from build123d import *

# Parameters (mm, degrees)
F1_DEPTH = 4.65
F2_R     = 1.75
F3_DEPTH = 13.001
F4_DEPTH = 2
F8_DEPTH = 12.5
F9_SIZE  = 0.99999
F10_R    = 0.5
F11_R    = 0.2
F12_W    = 7
F12_H    = 1.5


# Not quite as in the source:
# - a fillet or chamfer is up to 0.001 mm smaller than in the source, because OpenCascade refuses the exact size


with BuildPart() as f1:
    # F0 (on Front) → F1 (new body, symmetric)
    with BuildSketch(Plane.XZ):
        Polygon((23, 0), (0, 0), (0, -1.5), (0, -2), (-1.4, -2), (-1.4, -1.5), (-6, -1.5), (-6, -8.5), (-1.4, -8.5), (-1.4, -8), (0, -8), (0, -8.5), (0, -13), (1, -13), (8, -7), (23, -7), align=None)
    extrude(amount=F1_DEPTH, both=True)

    # F2 (on face) → F3 (cut, through all)
    with BuildSketch(Plane.XY):
        with Locations((18.4, 0)):
            Circle(F2_R)
    extrude(amount=-F3_DEPTH, mode=Mode.SUBTRACT)

    # F2 (on face) → F4 (cut)
    with BuildSketch(Plane.XY):
        Polygon((18.4, 3.2331615075), (15.6, 1.6165807537), (15.6, -1.6165807537), (18.4, -3.2331615075), (21.2, -1.6165807537), (21.2, 1.6165807537), align=None)
        with Locations((18.4, 0)):
            Circle(F2_R, mode=Mode.SUBTRACT)
    extrude(amount=-F4_DEPTH, mode=Mode.SUBTRACT)

    # F5 (on Front) → F6 (revolve, cut)
    with BuildSketch(Plane.XZ):
        Polygon((-6, -2.5), (-6, -5), (14, -5), (12.9, -3.9), (-4.6, -3.9), align=None)
    revolve(axis=Axis((22.399994296, 0, -5), (1, 0, 0)), mode=Mode.SUBTRACT)

    # F7 (on Front) → F8 (cut, symmetric)
    with BuildSketch(Plane.XZ):
        with BuildLine():
            ThreePointArc((4.1937742252, -5.4), (5.2054224947, -5.8762428879), (5.9, -5))
            ThreePointArc((5.9, -5), (5.2054224947, -4.1237571121), (4.1937742252, -4.6))
            ThreePointArc((4.1937742252, -4.6), (4.1, -5), (4.1937742252, -5.4))
        make_face()
        with BuildLine():
            ThreePointArc((4.1937742252, -5.4), (4.1, -5), (4.1937742252, -4.6))
            Line((4.1937742252, -4.6), (-6, -4.6))
            Line((-6, -4.6), (-6, -5.4))
            Line((-6, -5.4), (4.1937742252, -5.4))
        make_face()
    extrude(amount=F8_DEPTH, both=True, mode=Mode.SUBTRACT)

    # F9 (size 1 in the source; OpenCascade refuses exactly that, so slightly less here)
    f9_edges = [f1.edges().sort_by_distance(p)[0] for p in [
        (-6, 0, -8.5),
        (-6, 0, -1.5),
    ]]
    chamfer(f9_edges, length=F9_SIZE)

    # F10
    f10_edges = [f1.edges().sort_by_distance(p)[0] for p in [
        (0, 0, -2),
        (0, 0, -8),
    ]]
    fillet(f10_edges, radius=F10_R)

    # F11
    f11_edges = [f1.edges().sort_by_distance(p)[0] for p in [
        (-1.4, 0, -2),
        (-1.4, 0, -8),
    ]]
    fillet(f11_edges, radius=F11_R)

    # F12 (on Front) → F13 (revolve, cut)
    with BuildSketch(Plane.XZ):
        with Locations((-2.5, -4.25)):
            Rectangle(F12_W, F12_H)
    revolve(axis=Axis((4, 0, -5), (1, 0, 0)), mode=Mode.SUBTRACT)


solid = f1.part
Geometry: final body of the model. Coordinates: model frame, mm. A direction names the side the tool comes from. Give positions to 0.01 mm unless a question says otherwise; leave off trailing zeros. Write each loop counter-clockwise with the first axis right and the second up, starting at its lowest first coordinate (ties: lowest second). Pieces come first, ordered by that corner, then holes. Notation, with made-up numbers: (84, 59) -> (125, 59) arc R34 ccw to (125, 98) -> close; hole circle Ø10 at (57.25, 57). An arc over 180 degrees is marked (long way). Answer in a Markdown table with one row per item.
(1) Pin query (flat end, axial travel): pin 1 (4 mm diameter, centred on x = 6.5, y = 2, fed in from -Z); pin 2 (1.4 mm diameter, centred on x = 5, z = -5, fed in from +Y); pin 3 (0.6 mm diameter, centred on x = -0.5, y = -2, fed in from +Z); pin 4 (1.8 mm diameter, centred on x = 0, y = -3.5, fed in from +Z). Return the tip coordinate at first contact, or that it passes through.
Answers below:
| item | result |
|---|---|
| pin 1 | z = -10 |
| pin 2 | through |
| pin 3 | z = -1.9 |
| pin 4 | z = 0 |
(2) Ray query, line 1 along Y through (x, z) = (18.4, -5.2); line 2 along Z through (x, y) = (-0.75, 2.5); line 3 along Y through (x, z) = (9.5, -5). Return the intervals inside material, ascending. Write a range as [from, to].
Answers below:
| item | result |
|---|---|
| line 1 | [-4.65, -1.75], [1.75, 4.65] |
| line 2 | [-8, -5.4], [-4.6, -2] |
| line 3 | [-4.65, -1.1], [1.1, 4.65] |
(3) Set-up query: faces 4 (the flat face through (19.82, 2.414, -0.986)), 5 (the flat face through (-1, 3, -5.4)), 6 (the flat face through (1, 0, -3.7)), 7 (the flat face through (-3, 0, -8.5)). Return all of +Z, -Z, +X, -X, +Y, -Y with unobstructed straight access to the full face (end or side cutting, diameter ignored); none if empty.
Answers below:
| item | result |
|---|---|
| face 4 | +Z |
| face 5 | -X, +Y, -Y |
| face 6 | -X |
| face 7 | -Z, -X, +Y, -Y |
(4) Section query D-D on z = -9.25. Return loops of the section in (x, y) (3 decimals).
Answers below:
| item | result |
|---|---|
| outline | (0, -4.65) -> (5.375, -4.65) -> (5.375, 4.65) -> (0, 4.65) -> close |
(5) Section query C-C on x = 19.75. Return loops of the section in (y, z), then the cut area to 3 significant figures.
Answers below:
| item | result |
|---|---|
| outline | (-4.65, -7) -> (-1.11, -7) -> (-1.11, -2) -> (-2.45, -2) -> (-2.45, 0) -> (-4.65, 0) -> close; (1.11, -7) -> (4.65, -7) -> (4.65, 0) -> (2.45, 0) -> (2.45, -2) -> (1.11, -2) -> close |
| area | 44.1 mm^2 |
(6) Draft query along Z for faces 1 (the flat face through (-6, -2, -3)), 2 (the flat face through (0.5, -0.1, -13)), 3 (the cylindrical face through (-2, 0, -6.5)). Return one class per face: +Z half, -Z half, draft (parallel to the pull), parting line (faces both ways), or undercut.
Answers below:
| item | result |
|---|---|
| face 1 | draft |
| face 2 | -Z half |
| face 3 | undercut |
(7) Section query B-B on y = 3.75. Return loops of the section in (x, z).
Answers below:
| item | result |
|---|---|
| outline | (-6, -7.5) -> (-5, -8.5) -> (-1.4, -8.5) -> (-1.4, -8.2) arc R0.2 cw to (-1.2, -8) -> (-0.5, -8) arc R0.5 cw to (0, -8.5) -> (0, -13) -> (1, -13) -> (8, -7) -> (23, -7) -> (23, 0) -> (0, 0) -> (0, -1.5) arc R0.5 cw to (-0.5, -2) -> (-1.2, -2) arc R0.2 cw to (-1.4, -1.8) -> (-1.4, -1.5) -> (-5, -1.5) -> (-6, -2.5) -> (-6, -4.6) -> (4.19, -4.6) arc R0.9 cw (long way) to (4.19, -5.4) -> (-6, -5.4) -> close |
(8) Section query A-A on x = -2.25. Return loops of the section in (y, z).
Answers below:
| item | result |
|---|---|
| outline | (-4.65, -8.5) -> (4.65, -8.5) -> (4.65, -5.4) -> (1.45, -5.4) arc R1.5 cw to (-1.45, -5.4) -> (-4.65, -5.4) -> close; (-4.65, -4.6) -> (-1.45, -4.6) arc R1.5 cw to (1.45, -4.6) -> (4.65, -4.6) -> (4.65, -1.5) -> (-4.65, -1.5) -> close |
